For this review, take the finished solid that the model builds, in its own axes (mm). Face numbers are marked on the shaded views. A direction names the side the tool comes from. Coordinates: 2 decimals unless noted, no trailing zeros. Loops run counter-clockwise (first coordinate to the right, second up) from the corner with the lowest first, then second, coordinate; pieces in that order, holes last. Notation, with made-up numbers: (5.25, 65.5) -> (44.25, 65.5) arc R14 ccw to (44.25, 74.5) -> close; hole circle Ø8 at (-36, 54.5). An arc over 180 degrees is marked (long way). Answer in a Markdown table with one row per item.
from build123d import *

# Parameters (mm, degrees)
SKETCH_1_R          = 7
EXTRUDE_1_DEPTH     = 5.3
SKETCH_2_W          = 3.6
SKETCH_2_H          = 6
EXTRUDE_2_DEPTH     = 9.7
CUT_EXTRUDE_START   = -3.6
CUT_EXTRUDE_1_DEPTH = 3.6
CHAMFER_1_SIZE      = 1
SKETCH_4_R          = 1.5
EXTRUDE_3_DEPTH     = 2


# Read off the part's stored shape, not the designer's step: 切除-拉伸1
with BuildPart() as part:
    # 草图1 → 凸台-拉伸1 (new body)
    with BuildSketch(Plane.XY):
        Circle(SKETCH_1_R)
    extrude(amount=EXTRUDE_1_DEPTH)

    # 草图2 → 凸台-拉伸2 (add)
    with BuildSketch(Plane.XY.offset(5.3)):
        Rectangle(SKETCH_2_W, SKETCH_2_H)
    extrude(amount=EXTRUDE_2_DEPTH)

    # 切除-拉伸1 outline → 切除-拉伸1 (cut)
    with BuildSketch(Plane.ZY.offset(1.8).offset(CUT_EXTRUDE_START)):
        with BuildLine():
            Line((15, 3), (12, 3))
            ThreePointArc((12, 3), (14.121320344, 2.121320344), (15, 0))
            Line((15, 0), (15, 3))
        make_face()
        with BuildLine():
            Line((15, -3), (15, 0))
            ThreePointArc((15, 0), (14.121320344, -2.121320344), (12, -3))
            Line((12, -3), (15, -3))
        make_face()
    extrude(amount=CUT_EXTRUDE_1_DEPTH, mode=Mode.SUBTRACT)

    # 倒角1
    chamfer_1_edges = [part.edges().sort_by_distance(p)[0] for p in [
        (-7, 0, 0),
    ]]
    chamfer(chamfer_1_edges, length=CHAMFER_1_SIZE)

    # 草图4 → 凸台-拉伸3 (add)
    with BuildSketch(Plane.ZY.offset(1.8)):
        with Locations(Location((12, 0, 0), (0, 0, 180))):
            Circle(SKETCH_4_R)
    extrude_3 = extrude(amount=EXTRUDE_3_DEPTH)

    # 镜向1: 凸台-拉伸3 across plane
    add(extrude_3.mirror(Plane(origin=(0, 0, 0), x_dir=(0, 0, 1), z_dir=(1, 0, 0))))


solid = part.part
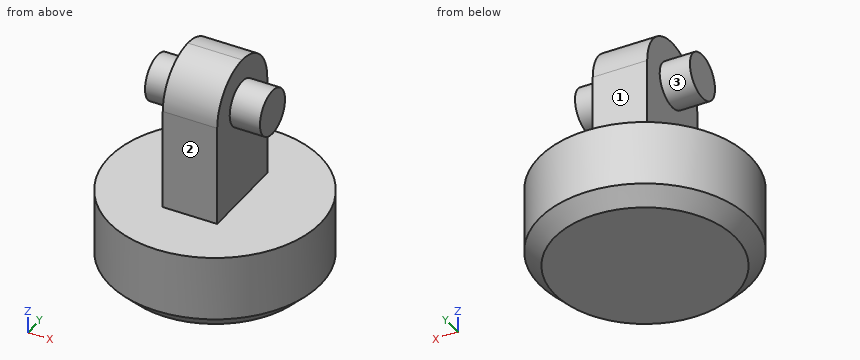
Item 1: Take a section at A-A, the plane x = 0. State the section outline as (y, z) points.
Worked answers:
| item | result |
|---|---|
| outline | (-7, 1) -> (-6, 0) -> (6, 0) -> (7, 1) -> (7, 5.3) -> (3, 5.3) -> (3, 12) arc R3 ccw to (-3, 12) -> (-3, 5.3) -> (-7, 5.3) -> close |
Item 2: For L1, parallel to Z at x = 4.5, y = -3; L2, parallel to X at y = -1.25, z = 10; L3, parallel to Z at x = 3.25, y = -1.25, list the stretches that pass through material, from the lowest coordinate up.
Worked answers:
| item | result |
|---|---|
| L1 | 0 to 5.3 |
| L2 | -1.8 to 1.8 |
| L3 | 0 to 5.3, 11.17 to 12.83 |
Item 3: Take a section at B-B, the plane z = 6. State the section outline as (x, y) points.
Worked answers:
| item | result |
|---|---|
| outline | (-1.8, -3) -> (1.8, -3) -> (1.8, 3) -> (-1.8, 3) -> close |
Item 4: For the marked faces 1, 2 and 3, list the 3-axis set-ups (+Z, -Z, +X, -X, +Y, -Y) from which the entire face can be reached by the end or side of a thin tool; tool diameter is ignored.
Worked answers:
| item | result |
|---|---|
| face 1 | +Z, +X, -X, +Y |
| face 2 | +Z, +X, -X, -Y |
| face 3 | -X |
Item 5: Take a section at C-C, the plane z = 11.25. State the section outline as (x, y) points.
Worked answers:
| item | result |
|---|---|
| outline | (-3.8, -1.3) -> (-1.8, -1.3) -> (-1.8, -3) -> (1.8, -3) -> (1.8, -1.3) -> (3.8, -1.3) -> (3.8, 1.3) -> (1.8, 1.3) -> (1.8, 3) -> (-1.8, 3) -> (-1.8, 1.3) -> (-3.8, 1.3) -> close |
Item 6: Insertion check: pin 1 (3 mm diameter, centred on x = 2, z = 10, fed in from -Y); pin 2 (3 mm diameter, centred on y = 0.5, z = 12, fed in from -X); pin 3 (3.5 mm diameter, centred on y = 0, z = 12, fed in from +X). Each pin has a flat end and moves straight along its axis. Give the tip position at first contact, or say it passes through.
Worked answers:
| item | result |
|---|---|
| pin 1 | y = -3 |
| pin 2 | x = -3.8 |
| pin 3 | x = 3.8 |
